Verification items for the finished model (mm, model axes). A direction names the side the tool comes from. Coordinates: 2 decimals unless noted, no trailing zeros. Write each loop counter-clockwise with the first axis right and the second up, starting at its lowest first coordinate (ties: lowest second). Pieces come first, ordered by that corner, then holes. Notation, with made-up numbers: (23, 79) -> (59, 79) arc R22 cw to (59, 101) -> close; hole circle Ø1 at (23, 34). An arc over 180 degrees is marked (long way). Answer in a Markdown table with one row per item.
```python
from build123d import *

# Parameters (mm, degrees)
F0_R      = 4.2926
F1_DEPTH  = 60.96
F2_R      = 1.2065
F3_DEPTH  = 2.413
F6_W      = 7.414472
F6_H      = 4.327964
F7_DEPTH  = 12.7
F8_R      = 2.54
F9_R      = 1.5875
F10_DEPTH = 6.457582


with BuildPart() as f1:
    # F0 (on Front) → F1 (new body)
    with BuildSketch(Plane.XZ):
        Circle(F0_R)
    extrude(amount=-F1_DEPTH)

    # F2 (on Front) → F3 (join)
    with BuildSketch(Plane.XZ):
        Circle(F2_R)
    extrude(amount=F3_DEPTH)

    # F4 (on Right) → F5 (revolve)
    with BuildSketch(Plane.YZ):
        with BuildLine():
            Line((-5.588, 0), (-2.413, 0))
            Line((-2.413, 0), (-2.413, 2.45745))
            add(Edge.make_bspline(
                [(-2.413, 2.45745), (-3.605465, 1.903019), (-5.753043, 0.65037), (-5.588, 0)],
                knots=[0, 0, 0, 0, 4.014933, 4.014933, 4.014933, 4.014933], degree=3))
        make_face()
    revolve(axis=Axis((0, -4.0005, 0), (0, 1, 0)))

    # F6 (on face) → F7 (join)
    with BuildSketch(Plane(origin=(0, 60.96, 0), x_dir=(-1, 0, 0), z_dir=(0, 1, 0))):
        Rectangle(F6_W, F6_H)
    extrude(amount=F7_DEPTH)

    # F8
    f8_edges = [f1.edges().sort_by_distance(p)[0] for p in [
        (-3.707236, 73.66, 0),
        (3.707236, 73.66, 0),
    ]]
    fillet(f8_edges, radius=F8_R)

    # F9 (on face) → F10 (cut, through all)
    with BuildSketch(Plane.XY.offset(2.163982)):
        with Locations((0, 67.818)):
            Circle(F9_R)
    extrude(amount=-F10_DEPTH, mode=Mode.SUBTRACT)


solid = f1.part
```
1. Thickness scan on line 1 (Y direction, x = 2, z = 2.5); line 2 (Z direction, x = 0.5, y = 63); line 3 (Y direction, x = 0, z = -0.85). Record the ranges inside material, lowest first. Write a range as from..to.
Geometry says:
| item | result |
|---|---|
| line 1 | 0..60.96 |
| line 2 | -2.16..2.16 |
| line 3 | -5.05..66.23, 69.41..73.66 |
2. Section check A-A, the plane y = 16. Record the boundary of the cut face in (x, z), plus the area to 3 significant figures.
Geometry says:
| item | result |
|---|---|
| outline | circle Ø8.59 at (0, 0) |
| area | 57.9 mm^2 |
3. Depth check by flat-ended pin: P1, Ø5, axis at x = 0, y = 67.818, coming from the -Z side; P2, Ø1.1, axis at x = -0.5, z = -3, coming from the +Y side; P3, Ø1.5, axis at x = 2, y = 18.5, coming from the +Z side. Enter the tip coordinate at first touch or a pass-through.
Geometry says:
| item | result |
|---|---|
| P1 | z = -2.16 |
| P2 | y = 60.96 |
| P3 | z = 4.11 |
4. Tool access check on faces 4 (the cylindrical face through (4.094, 30.053, 1.289)), 5 (the flat face through (0, 66, 2.164)), 6 (the flat face through (1, 0, -1)), 7 (the flat face through (-3.707, 66, 0)), 8 (the flat face through (3.707, 66, 0)). Record the directions out of +Z, -Z, +X, -X, +Y, -Y that give a thin tool (end or side, any length) a straight path to the whole face; none if there is none.
Geometry says:
| item | result |
|---|---|
| face 4 | +Y, -Y |
| face 5 | +Z, +X, -X, +Y |
| face 6 | none |
| face 7 | +Z, -Z, -X, +Y |
| face 8 | +Z, -Z, +X, +Y |
5. Mould release check, pull along Y, two halves, no side actions. Record for faces 1 (the flat face through (0, 60.96, -3)), 2 (the flat face through (0, 66, -2.164)), 3 (the cylindrical face through (-0.96, -1.19, -0.73)): released by +Y, released by -Y, zero draft, split by the parting line, or undercut.
Geometry says:
| item | result |
|---|---|
| face 1 | released by +Y |
| face 2 | zero draft |
| face 3 | undercut |
